Verification items for this drawing (mm, ordinates from the low corner). Give positions to 0.01 mm unless a question says otherwise; leave off trailing zeros. Loops run counter-clockwise (first coordinate to the right, second up) from the corner with the lowest first, then second, coordinate; pieces in that order, holes last. Notation, with made-up numbers: (-35.75, 71) -> (-28.75, 71) arc R29 ccw to (-28.75, 104) -> close; hole circle Ø1 at (0, -26). An arc over 180 degrees is marked (long way). Answer as a JSON object with one key per item and string values.
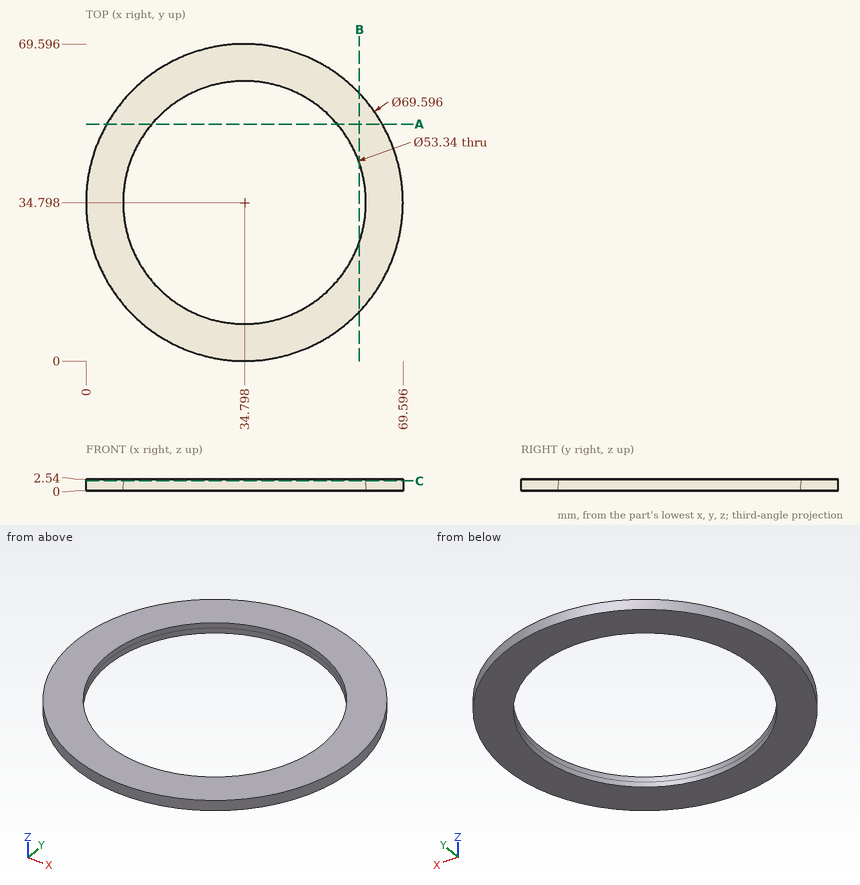
1) Depth check by flat-ended pin: P1, Ø1, axis at x = 27, z = 0.5, coming from the -Y side; P2, Ø1, axis at x = 52, z = 2, coming from the -Y side. Enter the tip coordinate at first touch or a pass-through.
Geometry check:
{"P1": "stops at y = 0.77", "P2": "stops at y = 4.27"}
2) Material ranges on line 1 along X through (y, z) = (34, 0.95); line 2 along Y through (x, z) = (13.5, 1.3); line 3 along Y through (x, z) = (51, 1.5), recorded low to high. Write a range as from..to.
Geometry check:
{"line 1": "x = 0.01..8.14, 61.46..69.59", "line 2": "y = 7.28..18.75, 50.85..62.32", "line 3": "y = 4..13.61, 55.98..65.59"}
3) Section check C-C on z = 2.15. Record the cut outline in (x, y).
Geometry check:
{"outline": "circle Ø69.6 at (34.8, 34.8); hole circle Ø53.34 at (34.8, 34.8)"}
4) Section check A-A on y = 52. Record the cut outline in (x, z), plus the area to 3 significant figures.
Geometry check:
{"outline": "(4.55, 0) -> (14.42, 0) -> (14.42, 2.54) -> (4.55, 2.54) -> close; (55.18, 0) -> (65.05, 0) -> (65.05, 2.54) -> (55.18, 2.54) -> close", "area": "50.1 mm2"}
5) Section check B-B on x = 60. Record the cut outline in (y, z).
Geometry check:
{"outline": "(10.8, 0) -> (26.07, 0) -> (26.07, 2.54) -> (10.8, 2.54) -> close; (43.52, 0) -> (58.79, 0) -> (58.79, 2.54) -> (43.52, 2.54) -> close"}
